Geometry: final body of the model. Coordinates: model frame, mm. A direction names the side the tool comes from. Give positions to 0.01 mm unless a question says otherwise; leave off trailing zeros. Write each loop counter-clockwise with the first axis right and the second up, starting at its lowest first coordinate (ties: lowest second). Pieces come first, ordered by that corner, then holes.
Q1. Section A-A (x = 0). Return the cut outline in (y, z).
Q2. Reachability of faces 1 (the flat face through (-10, 2.95, 36)), 2 (the flat face through (-33, -4, 109)), 3 (the flat face through (25, -7, 92)), 4 (the flat face through (33, -5, 102.447)) from +Z, -Z, +X, -X, +Y, -Y: full face, straight path, thin tool, end or side. Return the list, or none.
Q3. Section C-C (x = -26). Return the cut outline in (y, z), plus the area to 3 significant figures.
Q4. Line query: line 1 (Z direction, x = 32.5, y = -1.5); line 2 (X direction, y = -1.5, z = 100); line 3 (Y direction, x = -3, z = 85). Output: solid intervals per line, ascending.
Q5. Section B-B (z = 39). Return the cut outline in (x, y).
Q6. Mould query, pull axis X, two halves, no side actions, for faces 5 (the flat face through (35, 1, 105)), 6 (the flat face through (-29.5, -1, 109)), 7 (the flat face through (-32, -2, 117.985)). Classes: +X half, -X half, draft (parallel to the pull), parting line (faces both ways), or undercut.
Q7. Pin query (flat end, axial travel): pin 1 Ø1.3 at (y, z) = (-2.5, 111.5) entering from +X; pin 2 Ø2 at (x, z) = (-32, 101.5) entering from -Y; pin 3 Ø6 at (x, y) = (7.5, 3.5) entering from +Z. Return the tip coordinate at first contact, or that it passes through.
from build123d import *

# Parameters (mm, degrees)
BOSS_EXTRUDE4_DEPTH     = 5
SKETCH11_W              = 70
SKETCH11_H              = 5
BOSS_EXTRUDE5_DEPTH     = 40
FILLET1_R               = 10
FILLET2_R               = 10
SKETCH21_R              = 1.6
CUT_EXTRUDE1_DEPTH      = 131.853043071
CIRPATTERN1_COUNT       = 4
SKETCH22_R              = 2.86
CUT_EXTRUDE2_DEPTH      = 2.95
CIRPATTERN2_COUNT       = 4
FILLET4_R               = 2
SKETCH25_W              = 19
SKETCH25_H              = 10
BOSS_EXTRUDE6_DEPTH     = 4
CUT_EXTRUDE4_DEPTH      = 9.5
CUT_EXTRUDE4_DEPTH_BACK = 5.5
SKETCH26_W              = 11.1
SKETCH26_H              = 12
BOSS_EXTRUDE9_DEPTH     = 1.5
BOSS_EXTRUDE10_DEPTH    = 10
SKETCH35_W              = 10.92028557
SKETCH35_H              = 17.996185279
BOSS_EXTRUDE11_DEPTH    = 2.4
BOSS_EXTRUDE12_DEPTH    = 3
SKETCH37_R              = 1.05
CUT_EXTRUDE6_DEPTH      = 3
SKETCH39_R              = 1.65
CUT_EXTRUDE7_DEPTH      = 135.508959181
SKETCH40_W              = 4
SKETCH40_H              = 19
CUT_EXTRUDE8_DEPTH      = 5.5


with BuildPart() as part:
    # Sketch9 → Boss-Extrude4 (new body)
    with BuildSketch(Plane(origin=(0, 0, 0), x_dir=(1, 0, 0), z_dir=(0, 1, 0))):
        with BuildLine():
            Line((-35, -85.986185279), (35, -85.986185279))
            Line((35, -85.986185279), (16.969019665, -36.446473957))
            ThreePointArc((16.969019665, -36.446473957), (0, -5.285305191), (-16.969019665, -36.446473957))
            Line((-16.969019665, -36.446473957), (-35, -85.986185279))
        make_face()
    extrude(amount=BOSS_EXTRUDE4_DEPTH)

    # Sketch11 → Boss-Extrude5 (add)
    with BuildSketch(Plane.XY.offset(85.986185279)):
        with Locations((0, 2.5)):
            Rectangle(SKETCH11_W, SKETCH11_H)
    extrude(amount=BOSS_EXTRUDE5_DEPTH)

    # Fillet1
    fillet1_edges = [part.edges().sort_by_distance(p)[0] for p in [
        (-16.969019665, 2.5, 36.446473957),
    ]]
    fillet(fillet1_edges, radius=FILLET1_R)

    # Fillet2
    fillet2_edges = [part.edges().sort_by_distance(p)[0] for p in [
        (16.969019665, 2.5, 36.446473957),
    ]]
    fillet(fillet2_edges, radius=FILLET2_R)

    # Sketch21 → Cut-Extrude1 (cut, through all)
    with BuildSketch(Plane(origin=(0, 0, 0), x_dir=(-1, 0, 0), z_dir=(0, -1, 0))):
        with Locations(Location((8.838834765, -16.647350514, 0), (0, 0, 90))):
            Circle(SKETCH21_R)
    cut_extrude1 = extrude(amount=-CUT_EXTRUDE1_DEPTH, mode=Mode.SUBTRACT)

    # CirPattern1: Cut-Extrude1 ×4 about axis
    cirpattern1_axis = Axis((0, 0, 25.486185279), (0, 1, 0))
    for i in range(1, CIRPATTERN1_COUNT):
        add(cut_extrude1.rotate(cirpattern1_axis, i * 360 / CIRPATTERN1_COUNT), mode=Mode.SUBTRACT)

    # Sketch22 → Cut-Extrude2 (cut)
    with BuildSketch(Plane(origin=(0, 0, 0), x_dir=(-1, 0, 0), z_dir=(0, -1, 0))):
        with Locations(Location((8.838834765, -16.647350514, 0), (0, 0, 90))):
            Circle(SKETCH22_R)
    cut_extrude2 = extrude(amount=-CUT_EXTRUDE2_DEPTH, mode=Mode.SUBTRACT)

    # CirPattern2: Cut-Extrude2 ×4 about axis
    cirpattern2_axis = Axis((0, 0, 25.486185279), (0, 1, 0))
    for i in range(1, CIRPATTERN2_COUNT):
        add(cut_extrude2.rotate(cirpattern2_axis, i * 360 / CIRPATTERN2_COUNT), mode=Mode.SUBTRACT)

    # Fillet4
    fillet4_edges = [part.edges().sort_by_distance(p)[0] for p in [
        (35, 2.5, 125.986185279),
        (-35, 2.5, 125.986185279),
        (35, 2.5, 85.986185279),
        (-35, 2.5, 85.986185279),
    ]]
    fillet(fillet4_edges, radius=FILLET4_R)

    # Sketch25 → Boss-Extrude6 (add)
    with BuildSketch(Plane(origin=(-35, 0, -0.505457993), x_dir=(0, 0, -1), z_dir=(1, 0, 0))):
        with Locations((-108.99, -5)):
            Rectangle(SKETCH25_W, SKETCH25_H)
    extrude(amount=BOSS_EXTRUDE6_DEPTH)

    # Sketch26 → Cut-Extrude4 (cut, two sides: drawn at the far end of the back side and taken through both)
    with BuildSketch(Plane(origin=(-31, 0, -0.505457993), x_dir=(0, 0, -1), z_dir=(1, 0, 0)).offset(-CUT_EXTRUDE4_DEPTH_BACK)):
        with Locations((-108.99, -10)):
            Rectangle(SKETCH26_W, SKETCH26_H)
    extrude(amount=CUT_EXTRUDE4_DEPTH + CUT_EXTRUDE4_DEPTH_BACK, mode=Mode.SUBTRACT)

    # Sketch31 → Boss-Extrude9 (add)
    with BuildSketch(Plane(origin=(-31, 0, 0), x_dir=(0, 0, -1), z_dir=(1, 0, 0))):
        Polygon((-99.484542007, -4), (-102.934542007, -4), (-102.934542007, -4.5), (-98.984542007, -4.5), (-98.984542007, 0), (-117.984542007, 0), (-117.984542007, -4.5), (-114.034542007, -4.5), (-114.034542007, -4), (-117.484542007, -4), (-117.484542007, -2.4), (-99.484542007, -2.4), align=None)
    extrude(amount=BOSS_EXTRUDE9_DEPTH)

    # Sketch32 → Boss-Extrude10 (add)
    with BuildSketch(Plane.XZ):
        Polygon((31, 99.49), (31, 102.447343342), (35, 102.447343342), (35, 94.49), (20.07971443, 94.49), (11.750844515, 94.49), (11.750844515, 99.49), align=None)
        Polygon((31, 117.486185279), (31, 114.375323916), (35, 114.375323916), (35, 122.486185279), (20.07971443, 122.486185279), (11.750844515, 122.486185279), (11.750844515, 117.486185279), align=None)
    extrude(amount=BOSS_EXTRUDE10_DEPTH)

    # Sketch35 → Boss-Extrude11 (add)
    with BuildSketch(Plane(origin=(0, 0, 0), x_dir=(-1, 0, 0), z_dir=(0, -1, 0))):
        with Locations((-25.539857215, -108.48809264)):
            Rectangle(SKETCH35_W, SKETCH35_H)
    extrude(amount=BOSS_EXTRUDE11_DEPTH)

    # Sketch36 → Boss-Extrude12 (add)
    with BuildSketch(Plane.XZ.offset(10)):
        with BuildLine():
            ThreePointArc((22.024925014, 126.104087017), (24.995762953, 123.490002992), (27.97397303, 126.095684876))
            ThreePointArc((27.97397303, 126.095684876), (27.981571922, 126.293199831), (28, 126.49))
            ThreePointArc((28, 126.49), (25, 129.49), (22, 126.49))
            ThreePointArc((22, 126.49), (22.017642345, 126.297378059), (22.024925014, 126.104087017))
        make_face()
        with BuildLine():
            Line((18.846010194, 122.486185279), (31.109279434, 122.486185279))
            ThreePointArc((31.109279434, 122.486185279), (28.855912346, 123.695305938), (27.97397303, 126.095684876))
            ThreePointArc((27.97397303, 126.095684876), (24.995762953, 123.490002992), (22.024925014, 126.104087017))
            ThreePointArc((22.024925014, 126.104087017), (21.128493018, 123.68620066), (18.846010194, 122.486185279))
        make_face()
        with BuildLine():
            ThreePointArc((28, 90.49), (27.981571922, 90.686800169), (27.97397303, 90.884315124))
            ThreePointArc((27.97397303, 90.884315124), (24.995762953, 93.489997008), (22.024925014, 90.875912983))
            ThreePointArc((22.024925014, 90.875912983), (22.017642345, 90.682621941), (22, 90.49))
            ThreePointArc((22, 90.49), (25, 87.49), (28, 90.49))
        make_face()
        with BuildLine():
            ThreePointArc((27.97397303, 90.884315124), (28.855912346, 93.284694062), (31.109279434, 94.493814721))
            Line((31.109279434, 94.493814721), (18.846010194, 94.493814721))
            ThreePointArc((18.846010194, 94.493814721), (21.128493018, 93.29379934), (22.024925014, 90.875912983))
            ThreePointArc((22.024925014, 90.875912983), (24.995762953, 93.489997008), (27.97397303, 90.884315124))
        make_face()
    extrude(amount=-BOSS_EXTRUDE12_DEPTH)

    # Sketch37 → Cut-Extrude6 (cut)
    with BuildSketch(Plane(origin=(0, -10, 0), x_dir=(-1, 0, 0), z_dir=(0, -1, 0))):
        with Locations(Location((-25, -126.49, 0), (0, 0, 90))):
            Circle(SKETCH37_R)
        with Locations(Location((-25, -90.49, 0), (0, 0, 270))):
            Circle(SKETCH37_R)
    extrude(amount=-CUT_EXTRUDE6_DEPTH, mode=Mode.SUBTRACT)

    # Sketch39 → Cut-Extrude7 (cut, through all)
    with BuildSketch(Plane(origin=(0, 0, 0), x_dir=(-1, 0, 0), z_dir=(0, -1, 0))):
        with Locations(Location((0, -25.486185279, 0), (0, 0, 90))):
            Circle(SKETCH39_R)
    extrude(amount=-CUT_EXTRUDE7_DEPTH, mode=Mode.SUBTRACT)

    # Sketch40 → Cut-Extrude8 (cut)
    with BuildSketch(Plane(origin=(0, -10, 0), x_dir=(-1, 0, 0), z_dir=(0, -1, 0))):
        with Locations((33, -108.484542007)):
            Rectangle(SKETCH40_W, SKETCH40_H)
    extrude(amount=-CUT_EXTRUDE8_DEPTH, mode=Mode.SUBTRACT)


solid = part.part
Computed:
1. outline: (0, 5.29) - (5, 5.29) - (5, 23.84) - (0, 23.84) - close; (0, 27.14) - (5, 27.14) - (5, 125.99) - (0, 125.99) - close
2. face 1: -Y
2. face 2: +X, -X, -Y
2. face 3: -Z, +X, -X
2. face 4: +X, -Y
3. outline: (0, 61.26) - (5, 61.26) - (5, 125.99) - (0, 125.99) - close
3. area: 324 mm2
4. line 1: z = 94.49 to 102.45, 114.38 to 122.49
4. line 2: x = -35 to -29.5, 20.08 to 35
4. line 3: y = 0 to 5
5. outline: (-18.04, 0) - (18.04, 0) - (18.04, 5) - (-18.04, 5) - close
6. face 5: +X half
6. face 6: undercut
6. face 7: draft
7. pin 1: stops at x = 31
7. pin 2: stops at y = -4.5
7. pin 3: stops at z = 125.99
